Input: part model. Units: mm. Frame: model coordinates. A direction names the side the tool comes from. Round coordinates to 2 decimals unless told otherwise and drop trailing zeros. Order: outer loops, then holes, each group sorted by start corner. A loop starts at its lowest first (then second) coordinate and runs counter-clockwise, first axis right, second up. Notation, with made-up numbers: (22, 49.25) -> (44, 49.25) arc R22 cw to (44, 58.25) -> close; hole circle Ø11 at (-24, 19). An arc over 180 degrees is marked (long way). Answer as CSV lines item,"result". Start each with the question number.
1) Section query C-C, the plane y = 0. Output: boundary loops of the cut face in (x, z), and give its area (3 significant figures).
2) Section query D-D, the plane x = 1. Output: boundary loops of the cut face in (y, z), and give its area (3 significant figures).
3) Mould query, pull axis Z, two halves, no side actions, for faces 1 (the face through (0, -10, 1)), 2 (the face through (-29, 15, 3)), 3 (the face through (0, 15, 15)), 4 (the face through (-31.31, 14.52, 8.5)). Classes: +Z half, -Z half, draft (parallel to the pull), parting line (faces both ways), or undercut.
4) Section query B-B, the plane z = 7.5. Output: boundary loops of the cut face in (x, y).
5) Line query: L1, parallel to Y at x = -13.5, z = 1.7; L2, parallel to X at y = 0, z = 0.8; L3, parallel to Z at x = -30, y = 14.5. Output: solid intervals per line, ascending.
6) Section query A-A, the plane x = 30. Output: boundary loops of the cut face in (y, z).
7) Access query for faces 5 (the face through (5, 7.3, 1.5)), 6 (the face through (0, 13, 9)), 7 (the face through (0, 16, 7)). Directions: +Z, -Z, +X, -X, +Y, -Y. A direction counts if a zero-diameter tool reaches every point of the face in a straight line with its end or side. Return the directions, or none.
8) First-contact query: P1, Ø4, axis at x = -30, z = 7.5, coming from the -Y side; P2, Ø2.5, axis at x = 29, y = 15, coming from the -Z side; P3, Ø2.5, axis at x = 30, z = 7.5, coming from the -Y side; P4, Ø1.5, axis at y = 3, z = 1.5, coming from the -X side. Flat tips, straight axial feed; report the tip coordinate or a pass-through.
```python
from build123d import *

# Parameters (mm, degrees)
SKETCH_1_W          = 50
SKETCH_1_H          = 20
EXTRUDE_1_DEPTH     = 3
SKETCH_2_W          = 50
SKETCH_2_H          = 15
EXTRUDE_2_DEPTH     = 6
SKETCH_5_W          = 50
SKETCH_5_H          = 12
CUT_EXTRUDE_2_DEPTH = 3
SKETCH_6_W          = 8
SKETCH_6_H          = 12
SKETCH_6_R          = 1.65
EXTRUDE_3_DEPTH     = 3


with BuildPart() as part:
    # 草图1 → 凸台-拉伸1 (new body)
    with BuildSketch(Plane.XY):
        Rectangle(SKETCH_1_W, SKETCH_1_H)
        with BuildLine():
            Line((-5.208438024, 2.5), (5.208438024, 2.5))
            ThreePointArc((5.208438024, 2.5), (5.761208823, 2.666666667), (6.129722688, 3.111111111))
            ThreePointArc((6.129722688, 3.111111111), (21.5, 0), (6.129722688, -3.111111111))
            ThreePointArc((6.129722688, -3.111111111), (5.761208823, -2.666666667), (5.208438024, -2.5))
            Line((5.208438024, -2.5), (-5.208438024, -2.5))
            ThreePointArc((-5.208438024, -2.5), (-5.761208823, -2.666666667), (-6.129722688, -3.111111111))
            ThreePointArc((-6.129722688, -3.111111111), (-21.5, 0), (-6.129722688, 3.111111111))
            ThreePointArc((-6.129722688, 3.111111111), (-5.761208823, 2.666666667), (-5.208438024, 2.5))
        make_face(mode=Mode.SUBTRACT)
        with BuildLine():
            Line((3.25, 5.5), (-3.25, 5.5))
            ThreePointArc((-3.25, 5.5), (-5, 7.25), (-3.25, 9))
            Line((-3.25, 9), (3.25, 9))
            ThreePointArc((3.25, 9), (5, 7.25), (3.25, 5.5))
        make_face(mode=Mode.SUBTRACT)
    extrude(amount=EXTRUDE_1_DEPTH)

    # 草图2 → 凸台-拉伸2 (add)
    with BuildSketch(Plane(origin=(0, 10, 0), x_dir=(1, 0, 0), z_dir=(0, 1, 0))):
        with Locations((0, -7.5)):
            Rectangle(SKETCH_2_W, SKETCH_2_H)
    extrude(amount=EXTRUDE_2_DEPTH)

    # 草图5 → 切除-拉伸2 (cut)
    with BuildSketch(Plane.XZ.offset(-10)):
        with Locations((0, 9)):
            Rectangle(SKETCH_5_W, SKETCH_5_H)
    extrude(amount=-CUT_EXTRUDE_2_DEPTH, mode=Mode.SUBTRACT)

    # 草图6 → 凸台-拉伸3 (add)
    with BuildSketch(Plane(origin=(0, 16, 0), x_dir=(1, 0, 0), z_dir=(0, 1, 0))):
        with Locations((29, -9)):
            Rectangle(SKETCH_6_W, SKETCH_6_H)
        with Locations((30, -7.5)):
            Circle(SKETCH_6_R, mode=Mode.SUBTRACT)
        with Locations((-29, -9)):
            Rectangle(SKETCH_6_W, SKETCH_6_H)
        with Locations((-30, -7.5)):
            Circle(SKETCH_6_R, mode=Mode.SUBTRACT)
    extrude(amount=-EXTRUDE_3_DEPTH)


solid = part.part
```
Findings:
1,outline,"(-25, 0) -> (-21.5, 0) -> (-21.5, 3) -> (-25, 3) -> close; (21.5, 0) -> (25, 0) -> (25, 3) -> (21.5, 3) -> close"
1,area,"21.0 mm^2"
2,outline,"(-10, 0) -> (-2.5, 0) -> (-2.5, 3) -> (-10, 3) -> close; (2.5, 0) -> (5.5, 0) -> (5.5, 3) -> (2.5, 3) -> close; (9, 0) -> (16, 0) -> (16, 15) -> (13, 15) -> (13, 3) -> (9, 3) -> close"
2,area,"88.5 mm^2"
3,face 1,"draft"
3,face 2,"-Z half"
3,face 3,"+Z half"
3,face 4,"undercut"
4,outline,"(-33, 13) -> (-31.65, 13) -> (-31.65, 16) -> (-33, 16) -> close; (-28.35, 13) -> (28.35, 13) -> (28.35, 16) -> (-28.35, 16) -> close; (31.65, 13) -> (33, 13) -> (33, 16) -> (31.65, 16) -> close"
5,L1,"y = -10 to -8, 8 to 16"
5,L2,"x = -25 to -21.5, 21.5 to 25"
5,L3,"z = 3 to 5.85, 9.15 to 15"
6,outline,"(13, 3) -> (16, 3) -> (16, 5.85) -> (13, 5.85) -> close; (13, 9.15) -> (16, 9.15) -> (16, 15) -> (13, 15) -> close"
7,face 5,"+Z, -Z"
7,face 6,"+Z, +X, -X, -Y"
7,face 7,"+Z, -Z, +X, -X, +Y"
8,P1,"stops at y = 13"
8,P2,"stops at z = 3"
8,P3,"passes through"
8,P4,"stops at x = -25"
